from build123d import *


with BuildPart() as part:
    # Sweep1: sweep along a path in Sketch4
    with BuildLine(Plane.XY) as sweep1_path:
        CenterArc((0, 0), 2.5, 0, 360)
    # Sketch3 → Sweep1 (sweep)
    with BuildSketch(Plane(origin=(0, 0, 0), x_dir=(0, 0, -1), z_dir=(1, 0, 0))):
        Polygon((-0.505, 6.945), (0.495, 6.945), (0.495, 7.987), (5.044289322, 7.987), (5.115, 8.057710678), (5.115, 9.77), (2.817453163, 12.18689992), (0.275, 9.77), (0.265, 9.375), (-0.285, 9.375), (-0.285, 9.77), (-2.706694808, 12.191694808), (-5.125, 9.773389617), (-5.125, 8.057710678), (-5.054289322, 7.987), (-0.505, 7.987), align=None)
    sweep(path=sweep1_path.line)


solid = part.part
Check sheet for the modelled part. Datum: model origin and axes. Units: mm. A direction names the side the tool comes from. Round coordinates to 2 decimals unless told otherwise and drop trailing zeros. Order: outer loops, then holes, each group sorted by start corner. A loop starts at its lowest first (then second) coordinate and runs counter-clockwise, first axis right, second up.
Q1. Scan lines: L1, parallel to Y at x = 0, z = -0.1 (3 decimals); L2, parallel to Z at x = -3.5, y = 9 (3 decimals); L3, parallel to Y at x = 0, z = -1.9. Record each from-to range of solid material in increasing order.
Filled sheet:
L1: y = -9.375 to -6.945, 6.945 to 9.375
L2: z = -5.115 to -0.272, 0.285 to 5.125
L3: y = -11.31 to -7.99, 7.99 to 11.31
Q2. Cross-section at A-A, the plane z = -4. Enter the section's corners in (x, y).
Filled sheet:
outline: circle Ø21.89 at (0, 0); hole circle Ø15.97 at (0, 0)
Q3. Depth check by flat-ended pin: P1, Ø5, axis at x = -1, z = -2.5, coming from the -Y side; P2, Ø1.5, axis at x = 1.5, z = 1, coming from the -Y side; P3, Ø9.5, axis at x = 0, y = 0, coming from the -Z side; P4, Ø2, axis at y = -6, z = -4, coming from the -X side. Enter the tip coordinate at first touch or a pass-through.
Filled sheet:
P1: stops at y = -12.19
P2: stops at y = -11.14
P3: passes through
P4: stops at x = -10.51
Q4. Draft check along Y on faces 4 (the face through (-1.04, 7.92, -2.8)), 5 (the face through (9.463, 2.98, -4.971)). Enter one of: pulls with the +Y half, pulls with the -Y half, needs draft (parallel to the pull), parting line crosses it, or undercut.
Filled sheet:
face 4: undercut
face 5: parting line crosses it
Q5. Set-up check for faces 1 (the face through (-1.04, 7.92, 2.75)), 2 (the face through (8.94, 2.82, 0.01)), 3 (the face through (-1.51, -6.78, 0)): record each of +Z, -Z, +X, -X, +Y, -Y from which the full face is reachable in a straight line by a thin tool's end or side.
Filled sheet:
face 1: +Z
face 2: none
face 3: +Z, -Z
Q6. Cross-section at B-B, the plane z = -1. Enter the section's corners in (x, y).
Filled sheet:
outline: circle Ø20.92 at (0, 0); hole circle Ø15.97 at (0, 0)
